Part model, mm, in its own coordinate system. Coordinates: 2 decimals unless noted, no trailing zeros. Loops run counter-clockwise (first coordinate to the right, second up) from the corner with the lowest first, then second, coordinate; pieces in that order, holes last. Notation, with made-up numbers: (-29.5, 34.25) - (-14.5, 34.25) arc R24 ccw to (-14.5, 61.25) - close; hole circle Ø6 at (16, 47.5). An arc over 180 degrees is marked (long way). One line per question, with ' | ' between items. Start each with the question number.
from build123d import *

# Parameters (mm, degrees)
SKETCH1_W           = 54.92426628
SKETCH1_H           = 112.31
SKETCH1_R           = 1.6
BOSS_EXTRUDE1_DEPTH = 3
FILLET1_R           = 6
SKETCH2_W           = 21.1074
SKETCH2_H           = 7.874
SKETCH2_R           = 1.55575
BOSS_EXTRUDE2_DEPTH = 2
SKETCH2_4_R         = 1.55575
CUT_EXTRUDE1_DEPTH  = 4
FILLET2_R           = 1
FILLET3_R           = 0.5


with BuildPart() as part:
    # Sketch1 → Boss-Extrude1 (new body)
    with BuildSketch(Plane(origin=(0, 0, 0), x_dir=(1, 0, 0), z_dir=(0, 1, 0))):
        with Locations((-64.799805622, 36.959272125)):
            Rectangle(SKETCH1_W, SKETCH1_H)
        with Locations((-80.599805622, -16.191669117)):
            Circle(SKETCH1_R, mode=Mode.SUBTRACT)
        with Locations((-80.599805622, -9.791669117)):
            Circle(SKETCH1_R, mode=Mode.SUBTRACT)
        with Locations((-80.599805622, -3.391669117)):
            Circle(SKETCH1_R, mode=Mode.SUBTRACT)
        with Locations((-49.399805622, -3.391669117)):
            Circle(SKETCH1_R, mode=Mode.SUBTRACT)
        with Locations((-49.399805622, -9.791669117)):
            Circle(SKETCH1_R, mode=Mode.SUBTRACT)
        with Locations((-49.399805622, -16.191669117)):
            Circle(SKETCH1_R, mode=Mode.SUBTRACT)
        with Locations((-49.399805622, 90.110213368)):
            Circle(SKETCH1_R, mode=Mode.SUBTRACT)
        with Locations((-49.399805622, 83.710213368)):
            Circle(SKETCH1_R, mode=Mode.SUBTRACT)
        with Locations((-49.399805622, 77.310213368)):
            Circle(SKETCH1_R, mode=Mode.SUBTRACT)
        with Locations((-80.599805622, 77.310213368)):
            Circle(SKETCH1_R, mode=Mode.SUBTRACT)
        with Locations((-80.599805622, 83.710213368)):
            Circle(SKETCH1_R, mode=Mode.SUBTRACT)
        with Locations((-80.599805622, 90.110213368)):
            Circle(SKETCH1_R, mode=Mode.SUBTRACT)
    extrude(amount=BOSS_EXTRUDE1_DEPTH)

    # Fillet1
    fillet1_edges = [part.edges().sort_by_distance(p)[0] for p in [
        (-92.261938762, 1.5, -93.114272125),
        (-37.337672482, 1.5, -93.114272125),
        (-37.337672482, 1.5, 19.195727875),
        (-92.261938762, 1.5, 19.195727875),
    ]]
    fillet(fillet1_edges, radius=FILLET1_R)

    # Sketch2 → Boss-Extrude2 (add)
    with BuildSketch(Plane(origin=(0, 3, 0), x_dir=(1, 0, 0), z_dir=(0, 1, 0))):
        with Locations((-64.799805622, 33.022272125)):
            Rectangle(SKETCH2_W, SKETCH2_H)
        with Locations((-72.578555622, 31.720522125)):
            Circle(SKETCH2_R, mode=Mode.SUBTRACT)
        with Locations((-57.021525285, 31.719768414)):
            Circle(SKETCH2_R, mode=Mode.SUBTRACT)
    extrude(amount=BOSS_EXTRUDE2_DEPTH)

    # Sketch2<4> → Cut-Extrude1 (cut, through all)
    with BuildSketch(Plane(origin=(0, 3, 0), x_dir=(1, 0, 0), z_dir=(0, 1, 0))):
        with Locations((-72.578555622, 31.720522125)):
            Circle(SKETCH2_4_R)
        with Locations((-57.021525285, 31.719768414)):
            Circle(SKETCH2_4_R)
    extrude(amount=-CUT_EXTRUDE1_DEPTH, mode=Mode.SUBTRACT)

    # Fillet2
    fillet2_edges = [part.edges().sort_by_distance(p)[0] for p in [
        (-64.799805622, 3, -29.085272125),
        (-54.246105622, 3, -33.022272125),
        (-64.799805622, 3, -36.959272125),
        (-75.353505622, 3, -33.022272125),
    ]]
    fillet(fillet2_edges, radius=FILLET2_R)

    # Fillet3
    fillet3_edges = [part.edges().sort_by_distance(p)[0] for p in [
        (-64.799805622, 5, -36.959272125),
        (-75.353505622, 5, -33.022272125),
        (-64.799805622, 5, -29.085272125),
        (-54.246105622, 5, -33.022272125),
    ]]
    fillet(fillet3_edges, radius=FILLET3_R)


solid = part.part
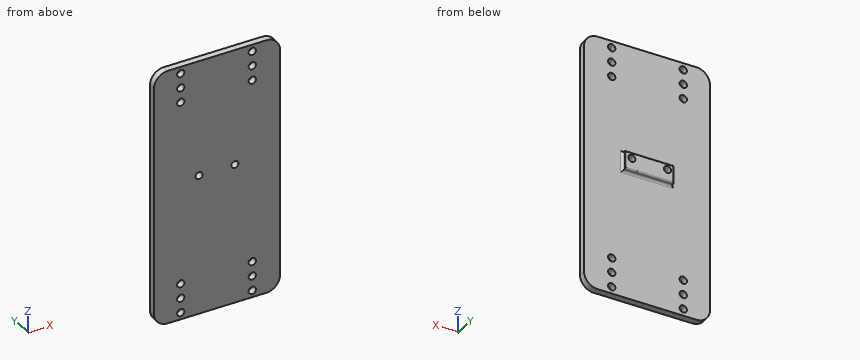
1) Pin check, flat tip, straight feed: pin 1 Ø12 at (x, z) = (-84.5, -70.5) entering from +Y. Stop position of the tip, or through.
2) Band-saw the part on A-A on x = -73. List the corners of the cut face in (y, z), then the cut area to 3 significant figures.
3) Band-saw the part on B-B on y = 1.25. Count the separate pieces of the cut face and the enclosed holes in it, then the cut area to 3 significant figures.
4) Band-saw the part on C-C on x = -67.5. List the corners of the cut face in (y, z).
5) Band-saw the part on D-D on z = 6. List the corners of the cut face in (x, y).
6) Wall check: line 1 along X through (y, z) = (1.95, -83.5); line 2 along X through (y, z) = (2.8, -33); line 3 along Y through (x, z) = (-84, -58). Give the ranges that are in metal, low to high. Write a range as [from, to].
Values found:
1) pin 1: y = 3
2) outline: (0, -93.11) - (3, -93.11) - (3, -37.96) arc R1 cw to (4, -36.96) - (4.5, -36.96) arc R0.5 ccw to (5, -36.46) - (5, -33.22) - (0, -33.22) - close; (0, -30.22) - (5, -30.22) - (5, -29.59) arc R0.5 ccw to (4.5, -29.09) - (4, -29.09) arc R1 cw to (3, -28.09) - (3, 19.2) - (0, 19.2) - close | area: 338 mm²
3) separate pieces: 1 | enclosed holes: 14 | area: 6,030 mm²
4) outline: (0, -93.11) - (3, -93.11) - (3, -37.96) arc R1 cw to (4, -36.96) - (4.5, -36.96) arc R0.5 ccw to (5, -36.46) - (5, -29.59) arc R0.5 ccw to (4.5, -29.09) - (4, -29.09) arc R1 cw to (3, -28.09) - (3, 19.2) - (0, 19.2) - close
5) outline: (-92.26, 0) - (-37.34, 0) - (-37.34, 3) - (-92.26, 3) - close
6) line 1: [-92.26, -82.19], [-79.01, -50.99], [-47.81, -37.34] | line 2: [-92.26, -73.46], [-71.69, -57.91], [-56.14, -37.34] | line 3: [0, 3]
